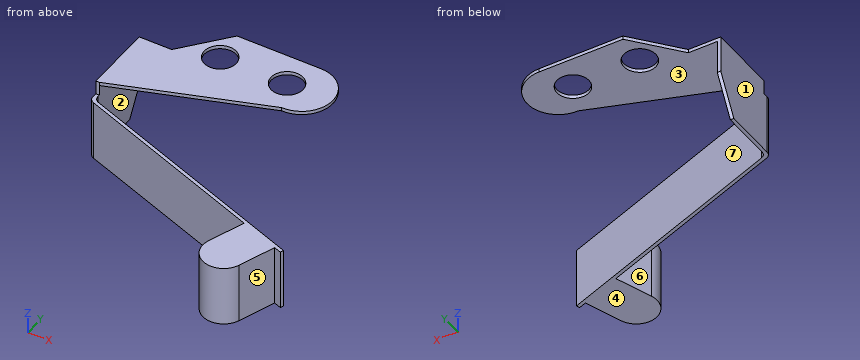
from build123d import *

# Parameters (mm, degrees)
EXTRUDE_1_DEPTH     = 5.33
SKETCH_3_W          = 18.524948115
SKETCH_3_H          = 1
CUT_EXTRUDE_2_DEPTH = 8
SKETCH_4_R          = 1.143
CUT_EXTRUDE_3_DEPTH = 8
SKETCH_5_W          = 14.906487706
SKETCH_5_H          = 5.08
CUT_EXTRUDE_4_DEPTH = 8.5
FILLET_1_R          = 0.5
SKETCH_6_W          = 1
SKETCH_6_H          = 0.794629951
CUT_EXTRUDE_5_DEPTH = 8.5
CUT_EXTRUDE_6_DEPTH = 8.5


with BuildPart() as part:
    # Эскиз1 → Бобышка-Вытянуть1 (new body)
    with BuildSketch(Plane.XY):
        with BuildLine():
            Line((-3.73172272, 3.969749711), (2.26827728, 3.969749711))
            ThreePointArc((2.26827728, 3.969749711), (4.49077728, 1.719238545), (2.212607957, -0.474901673))
            Line((2.212607957, -0.474901673), (-8.48172272, -4.233380934))
            Line((-8.48172272, -4.233380934), (-8.48172272, -4.745198404))
            Line((-8.48172272, -4.745198404), (8.926034324, -11.081103814))
            Line((8.926034324, -11.081103814), (8.840529289, -11.316026969))
            Line((8.840529289, -11.316026969), (8.31500946, -11.124753394))
            Line((8.31500946, -11.124753394), (7.374454066, -13.708908101))
            ThreePointArc((7.374454066, -13.708908101), (5.45188492, -14.605416817), (4.555376204, -12.682847671))
            Line((4.555376204, -12.682847671), (5.495931598, -10.098692964))
            Line((5.495931598, -10.098692964), (-8.73172272, -4.920250289))
            Line((-8.73172272, -4.920250289), (-8.73172272, 0.766619066))
            Line((-8.73172272, 0.766619066), (-6.416304518, 0.766619066))
            Line((-6.416304518, 0.766619066), (-3.73172272, 3.969749711))
        make_face()
    extrude(amount=EXTRUDE_1_DEPTH)

    # Эскиз3 → Вырез-Вытянуть2 (cut)
    with BuildSketch(Plane(origin=(-2.517250451, -6.916088773, 0), x_dir=(0.9396926207859082, -0.34202014332566943, 0), z_dir=(0.34202014332566943, 0.9396926207859082, 0))):
        with Locations((2.915215245, -4.83)):
            Rectangle(SKETCH_3_W, SKETCH_3_H)
    extrude(amount=-CUT_EXTRUDE_2_DEPTH, mode=Mode.SUBTRACT)

    # Эскиз4 → Вырез-Вытянуть3 (cut)
    with BuildSketch(Plane.XY.offset(5.33)):
        with Locations((-3.51932272, 1.683749711)):
            Circle(SKETCH_4_R)
        with Locations((1.25587728, 1.683749711)):
            Circle(SKETCH_4_R)
    extrude(amount=-CUT_EXTRUDE_3_DEPTH, mode=Mode.SUBTRACT)

    # Эскиз5 → Вырез-Вытянуть4 (cut)
    with BuildSketch(Plane(origin=(0, 3.969749711, 0), x_dir=(1, 0, 0), z_dir=(0, 1, 0))):
        with Locations((-1.028478867, -2.54)):
            Rectangle(SKETCH_5_W, SKETCH_5_H)
    extrude(amount=-CUT_EXTRUDE_4_DEPTH, mode=Mode.SUBTRACT)

    # Скругление1
    fillet_1_edges = [part.edges().sort_by_distance(p)[0] for p in [
        (-8.48172272, -4.745198404, 2.165),
        (-8.73172272, -4.920250289, 2.665),
    ]]
    fillet(fillet_1_edges, radius=FILLET_1_R)

    # Эскиз6 → Вырез-Вытянуть5 (cut)
    with BuildSketch(Plane(origin=(-8.48172272, 0, 0), x_dir=(0, 0, -1), z_dir=(1, 0, 0))):
        with Locations((-4.83, -4.630695909)):
            Rectangle(SKETCH_6_W, SKETCH_6_H)
    extrude(amount=-CUT_EXTRUDE_5_DEPTH, mode=Mode.SUBTRACT)

    # Эскиз7 → Вырез-Вытянуть6 (cut)
    with BuildSketch(Plane.ZY.offset(8.73172272)):
        Polygon((2.665, 0.766619066), (0, -0.740228), (0, 0.766619066), align=None)
    extrude(amount=-CUT_EXTRUDE_6_DEPTH, mode=Mode.SUBTRACT)


solid = part.part
Check sheet for the modelled part. Datum: model origin and axes. Units: mm. Face numbers are marked on the shaded views. A direction names the side the tool comes from. Round coordinates to 2 decimals unless told otherwise and drop trailing zeros. Order: outer loops, then holes, each group sorted by start corner. A loop starts at its lowest first (then second) coordinate and runs counter-clockwise, first axis right, second up. Notation, with made-up numbers: M -8.75,-19.75 L -4.75,-19.75 A9 ccw -4.75,-8.75 Z; hole C 81,34 d4. An arc over 180 degrees is marked long. One line per item, written item: value. Start each with the question number.
1. Section check B-B on x = -5.5. Enter the section's corners in (y, z).
2. Gauge pin test, flat ends, axial feed: P1, Ø2.5, axis at x = -3.52, y = 1.68, coming from the -Z side; P2, Ø3, axis at x = -5, y = -7.5, coming from the +Z side; P3, Ø1.9, axis at x = -8, z = 4, coming from the +Y side; P4, Ø2, axis at x = 1.26, y = 1.68, coming from the +Z side. Record the tip position at first contact, or that the pin passes through.
3. Access from +Z, -Z, +X, -X, +Y, -Y to the whole of each face (thin tool, end or side, straight path). Record for the marked faces 1, 2 and 3.
4. Section check C-C on z = 3.5. Enter the section's corners in (x, y) (3 decimals), and give its area (3 significant figures).
5. Release check for a two-part mould opening along Y. For the marked faces 4, 5, 6 and 7 record: released by +Y, released by -Y, zero draft, split by the parting line, or undercut.
6. Section check D-D on y = -3.25. Enter the section's corners in (x, z), and give its area (3 significant figures).
7. Scan lines: line 1 along X through (y, z) = (-2, 4.7); line 2 along Z through (x, y) = (-1, 0); line 3 along Y through (x, z) = (-3.75, 0.85). Record each from-to range of solid material in increasing order.
8. Section check A-A on y = 1.25. Enter the section's corners in (x, z), and give its area (3 significant figures).
Results found:
1. outline: M -6.1,0 L -5.83,0 L -5.83,4.33 L -6.1,4.33 Z; M -3.19,5.08 L 1.86,5.08 L 1.86,5.33 L -3.19,5.33 Z
2. P1: z = 5.08
2. P2: z = 4.33
2. P3: y = 0.77
2. P4: through
3. face 1: +Z, -Z, -X, +Y, -Y
3. face 2: -Z, +X, +Y
3. face 3: -Z, +X, +Y, -Y
4. outline: M -8.732,-4.57 A0.5 ccw -8.403,-5.04 L 5.496,-10.099 L 4.555,-12.683 A1.5 ccw 7.374,-13.709 L 8.315,-11.125 L 8.841,-11.316 L 8.926,-11.081 L -8.153,-4.865 A0.5 cw -8.482,-4.395 L -8.482,0.767 L -8.732,0.767 Z
4. area: 17.8 mm^2
5. face 4: zero draft
5. face 5: released by -Y
5. face 6: undercut
5. face 7: released by +Y
6. outline: M -8.73,0 L -8.48,0 L -8.48,5.08 L -5.68,5.08 L -5.68,5.33 L -8.73,5.33 Z
6. area: 2.03 mm^2
7. line 1: -8.73 to -8.48
7. line 2: 5.08 to 5.33
7. line 3: -6.73 to -6.47
8. outline: M -6.01,5.08 L -4.58,5.08 L -4.58,5.33 L -6.01,5.33 Z; M -2.46,5.08 L 0.2,5.08 L 0.2,5.33 L -2.46,5.33 Z; M 2.31,5.08 L 4.43,5.08 L 4.43,5.33 L 2.31,5.33 Z
8. area: 1.55 mm^2
